The listing builds one solid part. Answer for the finished solid, in the listing's coordinates (mm). Face numbers are marked on the shaded views. A direction names the side the tool comes from. Coordinates: 2 decimals unless noted, no trailing zeros. Order: outer loops, then holes, each group sorted by start corner. A loop starts at its lowest first (then second) coordinate and runs counter-clockwise, first axis right, second up. Notation, with made-up numbers: (1, 3) -> (33, 3) arc R19 cw to (33, 24) -> close; hole circle Ø8 at (-15.75, 10.5). An arc over 180 degrees is marked (long way). Answer in a Markdown table with one row per item.
```python
from build123d import *

# Parameters (mm, degrees)
BOSS_EXTRUDE1_DEPTH = 30
SKETCH2_R           = 1.275
CUT_EXTRUDE1_DEPTH  = 5


with BuildPart() as part:
    # Sketch1 → Boss-Extrude1 (new body)
    with BuildSketch(Plane.XY):
        Polygon((0, 0), (19.3, 0), (19.3, -1.2), (17.5, -1.2), (15.4, -2.4), (15.4, -4.4), (27.3, -4.4), (27.3, 3.175), (-27.3, 3.175), (-27.3, 0), (-20.9, 0), (-20.9, -7.5), (-15.9, -7.5), (-15.9, 0), align=None)
    extrude(amount=BOSS_EXTRUDE1_DEPTH)

    # Sketch2 → Cut-Extrude1 (cut)
    with BuildSketch(Plane.ZY.offset(20.9)):
        with Locations((7.5, -3.75)):
            Circle(SKETCH2_R)
        with Locations((22.5, -3.75)):
            Circle(SKETCH2_R)
    extrude(amount=-CUT_EXTRUDE1_DEPTH, mode=Mode.SUBTRACT)


solid = part.part
```
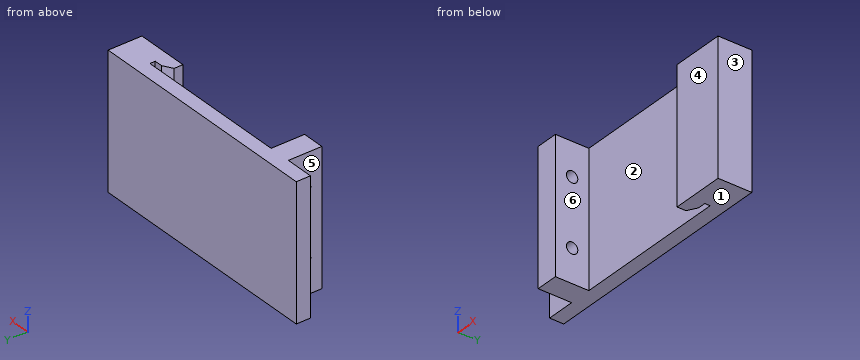
(1) Find the intervals of material crossed by line 1 along Y through (x, z) = (-16.95, 22.5) (3 decimals); line 2 along X through (y, z) = (-4, 18.5); line 3 along X through (y, z) = (-0.25, 9.5), in increasing order. Write a range as from..to.
Check values:
| item | result |
|---|---|
| line 1 | -7.5..-5.025, -2.475..3.175 |
| line 2 | -20.9..-15.9, 15.4..27.3 |
| line 3 | -20.9..-15.9, 19.3..27.3 |
(2) A cutting plane is placed at C-C, the plane z = 10.25. Determine the outline of the cut face in (x, y) (3 decimals).
Check values:
| item | result |
|---|---|
| outline | (-27.3, 0) -> (-20.9, 0) -> (-20.9, -7.5) -> (-15.9, -7.5) -> (-15.9, 0) -> (19.3, 0) -> (19.3, -1.2) -> (17.5, -1.2) -> (15.4, -2.4) -> (15.4, -4.4) -> (27.3, -4.4) -> (27.3, 3.175) -> (-27.3, 3.175) -> close |
(3) A cutting plane is placed at A-A, the plane y = -3.75. Determine the outline of the cut face in (x, z) (3 decimals), then the cut area to 4 significant figures.
Check values:
| item | result |
|---|---|
| outline | (-20.9, 0) -> (-15.9, 0) -> (-15.9, 6.225) -> (-20.9, 6.225) -> close; (-20.9, 8.775) -> (-15.9, 8.775) -> (-15.9, 21.225) -> (-20.9, 21.225) -> close; (-20.9, 23.775) -> (-15.9, 23.775) -> (-15.9, 30) -> (-20.9, 30) -> close; (15.4, 0) -> (27.3, 0) -> (27.3, 30) -> (15.4, 30) -> close |
| area | 481.5 mm² |
(4) A cutting plane is placed at B-B, the plane z = 22.5. Determine the outline of the cut face in (x, y) (3 decimals).
Check values:
| item | result |
|---|---|
| outline | (-27.3, 0) -> (-20.9, 0) -> (-20.9, -2.475) -> (-15.9, -2.475) -> (-15.9, 0) -> (19.3, 0) -> (19.3, -1.2) -> (17.5, -1.2) -> (15.4, -2.4) -> (15.4, -4.4) -> (27.3, -4.4) -> (27.3, 3.175) -> (-27.3, 3.175) -> close; (-20.9, -7.5) -> (-15.9, -7.5) -> (-15.9, -5.025) -> (-20.9, -5.025) -> close |
(5) Which of the six approach directions +Z, -Z, +X, -X, +Y, -Y give full straight-line access (tool end or side, diameter ignored) to the marked faces 4, 5 and 6?
Check values:
| item | result |
|---|---|
| face 4 | +Z, -Z, +X, -Y |
| face 5 | +Z, -Z, -X, -Y |
| face 6 | +Z, -Z, -Y |
(6) For a pull along X with two mould halves and no side action, classify the marked faces 1, 2 and 3 as released by +X, released by -X, zero draft, split by the parting line, or undercut.
Check values:
| item | result |
|---|---|
| face 1 | zero draft |
| face 2 | undercut |
| face 3 | released by +X |
(7) A cutting plane is placed at D-D, the plane x = 16. Determine the outline of the cut face in (y, z) (3 decimals).
Check values:
| item | result |
|---|---|
| outline | (-4.4, 0) -> (-2.057, 0) -> (-2.057, 30) -> (-4.4, 30) -> close; (0, 0) -> (3.175, 0) -> (3.175, 30) -> (0, 30) -> close |
(8) Flat-ended cylindrical pins translate along their axes: pin 1 (3 mm diameter, centred on x = -25, z = 8.5, fed in from -Y); pin 2 (4 mm diameter, centred on y = -5, z = 16.5, fed in from +X); pin 3 (13 mm diameter, centred on x = 20, z = 8.5, fed in from -Y); pin 4 (2 mm diameter, centred on y = -3.5, z = 19.5, fed in from -X). Find the tip coordinate at first contact, or state that the pin passes through.
Check values:
| item | result |
|---|---|
| pin 1 | y = 0 |
| pin 2 | x = 27.3 |
| pin 3 | y = -4.4 |
| pin 4 | x = -20.9 |
